Can you work these out from the model? Positions are in its coordinate system, mm. Round coordinates to 2 decimals unless told otherwise and drop trailing zeros. Loops run counter-clockwise (first coordinate to the right, second up) from the corner with the lowest first, then second, coordinate; pieces in that order, holes last. Notation, with made-up numbers: (17.25, 39.5) -> (55.25, 39.5) arc R25 ccw to (55.25, 73.5) -> close; hole circle Ø11 at (-38.75, -22.5). An arc over 180 degrees is marked (long way). Write item = value, one per line.
from build123d import *

# Parameters (mm, degrees)
ESQUISSE1_W                                       = 176
ESQUISSE1_H                                       = 118
BOSS_EXTRU_1_DEPTH                                = 8
ESQUISSE5_R                                       = 2.375000003
ESQUISSE5_R_2                                     = 1.250000003
ESQUISSE5_R_3                                     = 2.375
BOSS_EXTRU_2_DEPTH                                = 8
ESQUISSE6_R                                       = 2.375
ESQUISSE6_R_2                                     = 1.25
BOSS_EXTRU_3_DEPTH                                = 12
ESQUISSE8_R                                       = 2.375
ESQUISSE8_R_2                                     = 1.25
BOSS_EXTRU_4_DEPTH                                = 3
ESQUISSE16_W                                      = 18
ESQUISSE16_H                                      = 10
ENL_V_MAT_EXTRU_10_DEPTH                          = 221.800534301
ESQUISSE25_W                                      = 58.5
ESQUISSE25_H                                      = 15
ENL_V_MAT_EXTRU_17_DEPTH                          = 221.220062546
CHAMBRAGE_POUR_VIS_SIX_PANS_CREUX_M31_D           = 3.6
CHAMBRAGE_POUR_VIS_SIX_PANS_CREUX_M31_CBORE_D     = 6.5
CHAMBRAGE_POUR_VIS_SIX_PANS_CREUX_M31_CBORE_DEPTH = 3.4
SKETCH1_W                                         = 22.471601592
SKETCH1_H                                         = 9.999798569
CUT_EXTRUDE2_DEPTH                                = 10


with BuildPart() as part:
    # Esquisse1 → Boss.-Extru.1 (new body)
    with BuildSketch(Plane.XY):
        with Locations((-99.186852624, 56.386126343)):
            Rectangle(ESQUISSE1_W, ESQUISSE1_H)
    extrude(amount=BOSS_EXTRU_1_DEPTH)

    # Esquisse5 → Boss.-Extru.2 (add)
    # profile 1 of 4: a face of its own
    with BuildSketch(Plane.XY.offset(8)):
        with Locations((-22.394011126, 103.894915048)):
            Circle(ESQUISSE5_R)
        with Locations((-22.394011126, 103.894915048)):
            Circle(ESQUISSE5_R_2, mode=Mode.SUBTRACT)
    # profile 2 of 4: a face of its own
    with BuildSketch(Plane.XY.offset(8)):
        with Locations((-43.984011126, 88.654915048)):
            Circle(ESQUISSE5_R_3)
        with Locations((-43.984011126, 88.654915048)):
            Circle(ESQUISSE5_R_2, mode=Mode.SUBTRACT)
    # profile 3 of 4: a face of its own
    with BuildSketch(Plane.XY.offset(8)):
        with Locations((-43.984011126, 103.894915048)):
            Circle(ESQUISSE5_R_3)
        with Locations((-43.984011126, 103.894915048)):
            Circle(ESQUISSE5_R_2, mode=Mode.SUBTRACT)
    # profile 4 of 4: a face of its own
    with BuildSketch(Plane.XY.offset(8)):
        with Locations((-22.394011126, 88.654915048)):
            Circle(ESQUISSE5_R_3)
        with Locations((-22.394011126, 88.654915048)):
            Circle(ESQUISSE5_R_2, mode=Mode.SUBTRACT)
    extrude(amount=BOSS_EXTRU_2_DEPTH)

    # Esquisse6 → Boss.-Extru.3 (add)
    # profile 1 of 4: a face of its own
    with BuildSketch(Plane.XY.offset(8)):
        with Locations((-179.187599449, 33.468198675)):
            Circle(ESQUISSE6_R)
        with Locations((-179.187599449, 33.468198675)):
            Circle(ESQUISSE6_R_2, mode=Mode.SUBTRACT)
    # profile 2 of 4: a face of its own
    with BuildSketch(Plane.XY.offset(8)):
        with Locations((-121.10208697, 33.467532232)):
            Circle(ESQUISSE6_R)
        with Locations((-121.10208697, 33.467532232)):
            Circle(ESQUISSE6_R_2, mode=Mode.SUBTRACT)
    # profile 3 of 4: a face of its own
    with BuildSketch(Plane.XY.offset(8)):
        with Locations((-179.630514203, 82.466196864)):
            Circle(ESQUISSE6_R)
        with Locations((-179.630514203, 82.466196864)):
            Circle(ESQUISSE6_R_2, mode=Mode.SUBTRACT)
    # profile 4 of 4: a face of its own
    with BuildSketch(Plane.XY.offset(8)):
        with Locations((-121.545001725, 82.465530421)):
            Circle(ESQUISSE6_R)
        with Locations((-121.545001725, 82.465530421)):
            Circle(ESQUISSE6_R_2, mode=Mode.SUBTRACT)
    extrude(amount=BOSS_EXTRU_3_DEPTH)

    # Esquisse8 → Boss.-Extru.4 (add)
    # profile 1 of 4: a face of its own
    with BuildSketch(Plane.XY.offset(8)):
        with Locations((-18.201902813, 11.077271698)):
            Circle(ESQUISSE8_R)
        with Locations((-18.201902813, 11.077271698)):
            Circle(ESQUISSE8_R_2, mode=Mode.SUBTRACT)
    # profile 2 of 4: a face of its own
    with BuildSketch(Plane.XY.offset(8)):
        with Locations((-66.241902813, 11.077271698)):
            Circle(ESQUISSE8_R)
        with Locations((-66.241902813, 11.077271698)):
            Circle(ESQUISSE8_R_2, mode=Mode.SUBTRACT)
    # profile 3 of 4: a face of its own
    with BuildSketch(Plane.XY.offset(8)):
        with Locations((-66.241902813, 53.147271698)):
            Circle(ESQUISSE8_R)
        with Locations((-66.241902813, 53.147271698)):
            Circle(ESQUISSE8_R_2, mode=Mode.SUBTRACT)
    # profile 4 of 4: a face of its own
    with BuildSketch(Plane.XY.offset(8)):
        with Locations((-18.201902813, 53.147271698)):
            Circle(ESQUISSE8_R)
        with Locations((-18.201902813, 53.147271698)):
            Circle(ESQUISSE8_R_2, mode=Mode.SUBTRACT)
    extrude(amount=BOSS_EXTRU_4_DEPTH)

    # Esquisse16 → Enlèv. mat.-Extru.10 (cut, through all)
    with BuildSketch(Plane(origin=(0, 0, 0), x_dir=(-1, 0, 0), z_dir=(0, 0, -1))):
        with Locations((79.109390261, 9.929756241)):
            Rectangle(ESQUISSE16_W, ESQUISSE16_H)
        with Locations((119.580991853, 9.92955481)):
            Rectangle(ESQUISSE16_W, ESQUISSE16_H)
    extrude(amount=-ENL_V_MAT_EXTRU_10_DEPTH, mode=Mode.SUBTRACT)

    # Esquisse25 → Enlèv. mat.-Extru.17 (cut, through all)
    with BuildSketch(Plane.XY.offset(8)):
        with Locations((-99.186852624, 99.756126343)):
            Rectangle(ESQUISSE25_W, ESQUISSE25_H)
    extrude(amount=-ENL_V_MAT_EXTRU_17_DEPTH, mode=Mode.SUBTRACT)

    # Chambrage pour vis à six pans creux M31 (through all)
    with Locations(Plane.XY.offset(8)):
        with Locations((-99.186852624, 111.386126343), (-99.186852624, 1.386126343)):
            CounterBoreHole(CHAMBRAGE_POUR_VIS_SIX_PANS_CREUX_M31_D / 2, CHAMBRAGE_POUR_VIS_SIX_PANS_CREUX_M31_CBORE_D / 2, CHAMBRAGE_POUR_VIS_SIX_PANS_CREUX_M31_CBORE_DEPTH)

    # Sketch1 → Cut-Extrude2 (cut)
    with BuildSketch(Plane.XY.offset(8)):
        with Locations((-99.345191057, 9.929655526)):
            Rectangle(SKETCH1_W, SKETCH1_H)
    extrude(amount=-CUT_EXTRUDE2_DEPTH, mode=Mode.SUBTRACT)


solid = part.part
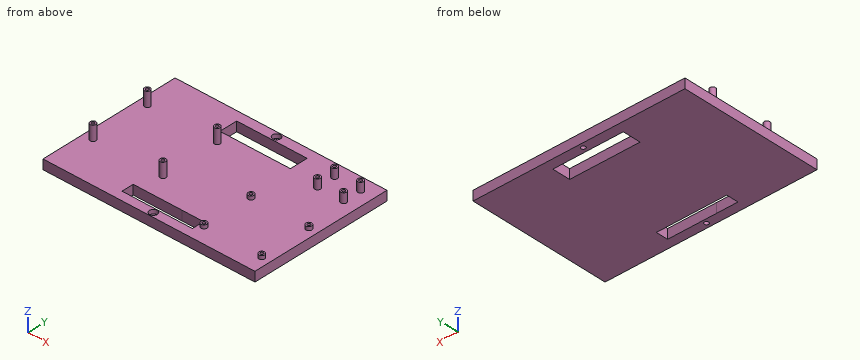
1. Suppose I cut it at B-B, the plane y = 58. List the corners of the cut face in (x, z) for me.
Entries:
outline = (-187.19, 0) -> (-11.19, 0) -> (-11.19, 8) -> (-187.19, 8) -> close
2. Suppose I cut it at C-C, the plane x = -136.5. List the corners of the cut face in (y, z) for me, and give its area (3 significant figures).
Entries:
outline = (-2.61, 0) -> (115.39, 0) -> (115.39, 8) -> (-2.61, 8) -> close
area = 944 mm²
3. Suppose I cut it at A-A, the plane z = 18. List the corners of the cut face in (x, y) for me (3 decimals), and give its area (3 significant figures).
Entries:
outline = circle Ø4.75 at (-179.631, 82.466); circle Ø4.75 at (-179.188, 33.468); circle Ø4.75 at (-121.545, 82.466); circle Ø4.75 at (-121.102, 33.468); hole circle Ø2.5 at (-179.631, 82.466); hole circle Ø2.5 at (-179.188, 33.468); hole circle Ø2.5 at (-121.545, 82.466); hole circle Ø2.5 at (-121.102, 33.468)
area = 51.2 mm²
4. I'm going to push flat-ended pins straight in: pin 1 (1 mm diameter, centred on x = -52, y = 23.5, fed in from +Z); pin 2 (1.5 mm diameter, centred on x = -41.5, z = 9, fed in from -Y); pin 3 (4 mm diameter, centred on x = -99.19, y = 111.39, fed in from +Z). Where does each tip first touch, or does it pass through?
Entries:
pin_1 = 8
pin_2 = 87.03
pin_3 = 4.6
5. I need wall thicknesses on line 1 (X direction, y = 9, z = 7.75); line 2 (Z direction, x = -172, y = 47.5); line 3 (X direction, y = 106, z = 9). Which ranges of each line are inside material? Lowest first, please. Write a range as [from, to].
Entries:
line_1 = [-187.19, -128.58], [-70.11, -11.19]
line_2 = [0, 8]
line_3 = [-45.08, -42.88], [-23.49, -21.29]
